Check sheet for the modelled part. Datum: model origin and axes. Units: mm. Face numbers are marked on the shaded views. A direction names the side the tool comes from. Round coordinates to 2 decimals unless told otherwise and drop trailing zeros. Write each loop counter-clockwise with the first axis right and the second up, starting at its lowest first coordinate (ties: lowest second). Pieces come first, ordered by that corner, then holes. Notation, with made-up numbers: (54, -37.75) - (76, -37.75) arc R21 cw to (76, -11.75) - close; hole circle Ø6 at (33, 64). An arc over 180 degrees is marked (long way). Use one line per item in the form item = value. Start each with the question number.
1) Section check D-D (x = 10.5). Record the boundary of the cut face in (y, z) (3 decimals).
2) Scan lines: probe 1 along Y at (x, z) = (19.5, -84) (3 decimals); probe 2 along X at (y, z) = (30.95, -38.1) (3 decimals); probe 3 along Y at (x, z) = (2.4, -114.3). Record each from-to range of solid material in increasing order.
3) Section check B-B (x = 27). Record the boundary of the cut face in (y, z) (3 decimals).
4) Gauge pin test, flat ends, axial feed: P1, Ø6, axis at x = 14, z = -75.5, coming from the -Y side; P2, Ø7.5, axis at y = 15.875, z = -139.7, coming from the +X side (3 decimals). Record the tip position at first contact, or that the pin passes through.
5) Set-up check for the marked faces 1 and 2: record each of +Z, -Z, +X, -X, +Y, -Y from which the full face is reachable in a straight line by a thin tool's end or side.
6) Section check A-A (z = -63.5). Record the boundary of the cut face in (x, y) (3 decimals), then the cut area to 3 significant figures.
7) Draft check along Y on the marked faces 3, 4 and 5. Enter one of: +Y half, -Y half, draft (parallel to the pull), parting line (faces both ways), or undercut.
8) Section check C-C (z = -43.5). Record the boundary of the cut face in (x, y) (3 decimals).
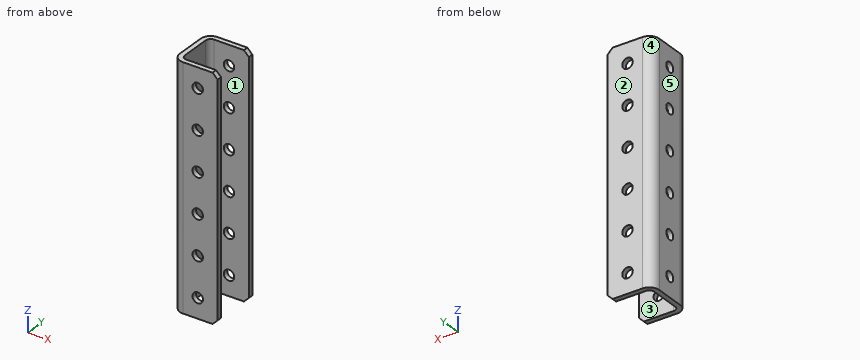
Autodesk Inventor part; units mm, degrees
ref_plane "YZ Plane" through (0, 0, 0) normal (1, 0, 0) x (0, 1, 0)
ref_plane "XZ Plane" through (0, 0, 0) normal (0, 1, 0) x (-1, 0, 0)
ref_plane "XY Plane" through (0, 0, 0) normal (0, 0, 1) x (1, 0, 0)
sketch "Sketch1" plane through (0, 0, 0) normal (0, 0, 1) x (1, 0, 0)
  line L0 (6.35, 28.575) -> (25.4, 28.575)
  line L1 (6.35, 31.75) -> (25.4, 31.75)
  line L2 (25.4, 0) -> (6.35, 0)
  arc A0 (0, 6.35) -> (6.35, 0) centre (6.35, 6.35) ccw
  line L3 (0, 6.35) -> (0, 25.4)
  arc A1 (6.35, 31.75) -> (0, 25.4) centre (6.35, 25.4) ccw
  line L4 (6.35, 31.75) -> (25.4, 31.75)
  line L5 (25.4, 28.575) -> (6.35, 28.575)
  arc A2 (6.35, 28.575) -> (3.175, 25.4) centre (6.35, 25.4) ccw
  line L6 (3.175, 25.4) -> (3.175, 6.35)
  arc A3 (3.175, 6.35) -> (6.35, 3.175) centre (6.35, 6.35) ccw
  line L7 (6.35, 3.175) -> (25.4, 3.175)
  line L8 (28.575, 3.175) -> (28.575, 0)
  line L9 (25.4, 31.75) -> (28.575, 31.75)
  line L10 (28.575, 28.575) -> (25.4, 28.575)
  line L11 (28.575, 31.75) -> (28.575, 28.575)
  line L12 (28.575, 0) -> (25.4, 0)
  line L13 (28.575, 3.175) -> (28.575, 0)
  line L14 (25.4, 3.175) -> (28.575, 3.175)
  point P0 (0, 0)
extrude "Extrusion1" add sketch "Sketch1" against normal blind 152.4
chamfer "Chamfer1" distance 3.175 angle 45 4 edges at (28.575, 30.1625, 0) (28.575, 1.5875, 0) (28.575, 30.1625, -152.4) (28.575, 1.5875, -152.4)
sketch "Sketch2" plane through (6.35, 31.75, 0) normal (0, 1, 0) x (1, 0, 0)
  line L0 (19.05, 0) -> (0, 0)
  line L1 (22.225, 3.175) -> (22.225, 149.225)
  point P0 (-6.35, 0)
  point P1 (9.525, 12.7)
  dimension "d5" = 12.7
  dimension "d6" = 12.7
hole "Hole1" at (15.875, 31.75, -12.7) direction (0, -1, 0) diameter 6.7056 end through all
pattern_linear "Rectangular Pattern1" count 6 spacing 25.4 along (0, 0, -1) of "Hole1"
hole "Hole2" at (0, 15.875, -12.7) direction (1, 0, 0) diameter 6.35 end through all
pattern_linear "Rectangular Pattern2" count 6 spacing 25.4 along (0, 0, -1) of "Hole2"
properties part number "DBK_C-Channel_6" material "Aluminum 6061"
Results are:
q1.outline = (0, -152.4) - (3.175, -152.4) - (3.175, 0) - (0, 0) - close; (28.575, -152.4) - (31.75, -152.4) - (31.75, 0) - (28.575, 0) - close
q2.probe_1 = 0 to 3.175, 28.575 to 31.75
q2.probe_2 = 3.265 to 12.522, 19.228 to 28.575
q2.probe_3 = 1.38 to 12.7, 19.05 to 30.37
q3.outline = (0, -150.8) - (3.175, -150.8) - (3.175, -1.6) - (0, -1.6) - close; (28.575, -150.8) - (31.75, -150.8) - (31.75, -1.6) - (28.575, -1.6) - close
q4.P1 = 0
q4.P2 = 3.175
q5.face_1 = +Z, -Z, +X
q5.face_2 = +Z, -Z, +X, -X, +Y
q6.outline = (0, 6.35) arc R6.35 ccw to (6.35, 0) - (12.522, 0) - (12.522, 3.175) - (6.35, 3.175) arc R3.175 cw to (3.175, 6.35) - (3.175, 12.7) - (0, 12.7) - close; (0, 19.05) - (3.175, 19.05) - (3.175, 25.4) arc R3.175 cw to (6.35, 28.575) - (12.522, 28.575) - (12.522, 31.75) - (6.35, 31.75) arc R6.35 ccw to (0, 25.4) - close; (19.228, 0) - (28.575, 0) - (28.575, 3.175) - (19.228, 3.175) - close; (19.228, 28.575) - (28.575, 28.575) - (28.575, 31.75) - (19.228, 31.75) - close
q6.area = 186 mm²
q7.face_3 = undercut
q7.face_4 = +Y half
q7.face_5 = draft
q8.outline = (0, 6.35) arc R6.35 ccw to (6.35, 0) - (28.575, 0) - (28.575, 3.175) - (6.35, 3.175) arc R3.175 cw to (3.175, 6.35) - (3.175, 25.4) arc R3.175 cw to (6.35, 28.575) - (28.575, 28.575) - (28.575, 31.75) - (6.35, 31.75) arc R6.35 ccw to (0, 25.4) - close
